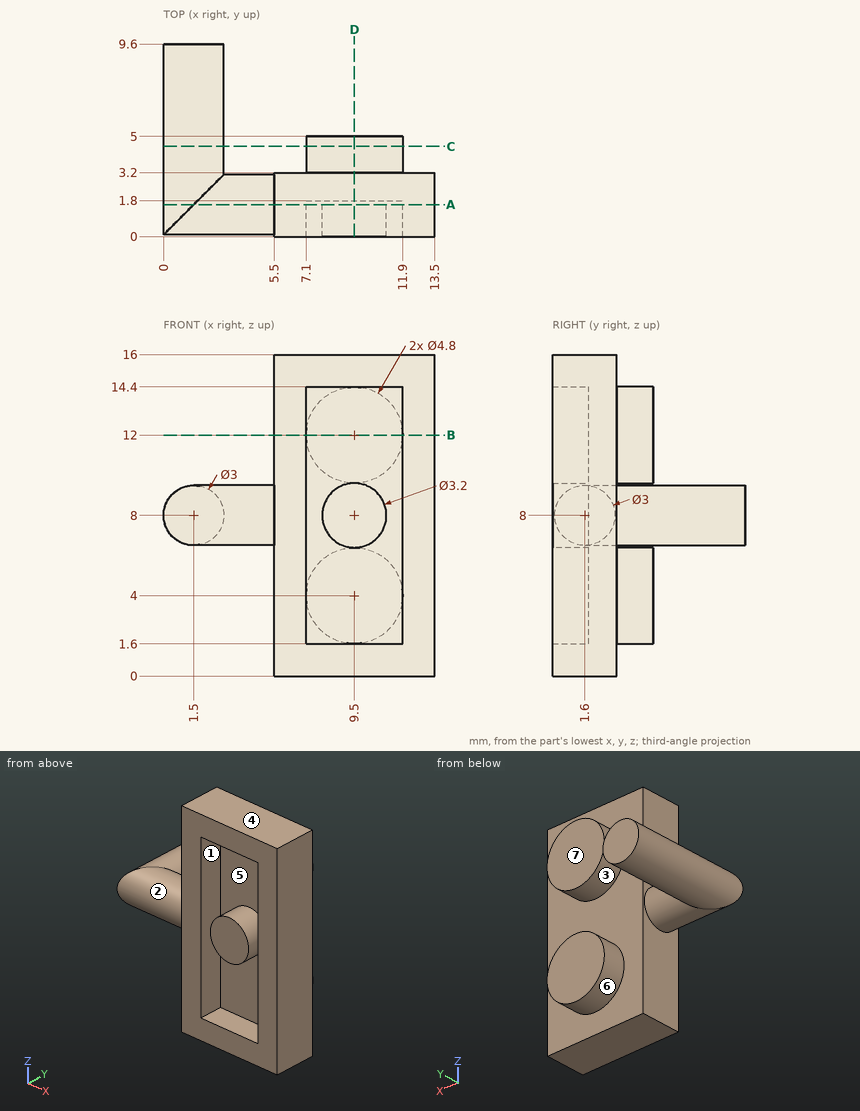
The drawing under review shows one solid part. Ordinate dimensions are in mm from its lowest x, y, z. A direction names the side the tool comes from. Round coordinates to 2 decimals unless told otherwise and drop trailing zeros. Loops run counter-clockwise (first coordinate to the right, second up) from the corner with the lowest first, then second, coordinate; pieces in that order, holes last. Notation, with made-up numbers: (61, -16) - (74, -16) arc R17 cw to (74, 3) - close; hole circle Ø5 at (-10.5, -18). An arc over 180 degrees is marked (long way). Put each result on its own line as item: value. Start each with the question number.
1. For the marked faces 5, 6 and 7, list the 3-axis set-ups (+Z, -Z, +X, -X, +Y, -Y) from which the entire face can be reached by the end or side of a thin tool; tool diameter is ignored.
2. Insertion check: P1, Ø1, axis at x = 4, z = 8.5, coming from the +Y side; P2, Ø1, axis at x = 3.5, z = 5.5, coming from the -Y side; P3, Ø4, axis at x = 5, z = 11, coming from the -Y side; P4, Ø2.5, axis at x = 10, z = 12, coming from the +Y side. Each pin has a flat end and moves straight along its axis. Give the tip position at first contact, or say it passes through.
3. Consider section C-C on y = 4.5. State the section outline as (x, z) points, plus the area to 3 significant figures.
4. Mouldability with a two-part tool opening along X and no side actions: class the marked faces 1, 2, 3 and 4 as +X half, -X half, draft (parallel to the pull), parting line (faces both ways), or undercut.
5. Consider section A-A on y = 1.6. State the section outline as (x, z) points.
6. Consider section B-B on z = 12. State the section outline as (x, y) points, plus the area to 3 significant figures.
7. Consider section D-D on x = 9.5. State the section outline as (y, z) points.
8. For probe 1 along Z at (x, y) = (10, 1.5); probe 2 along Y at (x, z) = (7, 10); probe 3 along X at (y, z) = (3, 4.5), list the stretches that pass through material, from the lowest coordinate up. Write a range as [from, to].
Result sheet:
1. face 5: -Y
1. face 6: +Y
1. face 7: +Z, -Z, +X, -X, +Y
2. P1: y = 3.1
2. P2: through
2. P3: y = 0
2. P4: y = 5
3. outline: circle Ø3 at (1.5, 8); circle Ø4.8 at (9.5, 4); circle Ø4.8 at (9.5, 12)
3. area: 43.3 mm^2
4. face 1: undercut
4. face 2: undercut
4. face 3: parting line
4. face 4: draft
5. outline: (1.5, 6.5) - (5.5, 6.5) - (5.5, 0) - (13.5, 0) - (13.5, 16) - (5.5, 16) - (5.5, 9.5) - (1.5, 9.5) arc R1.5 ccw to start; circle Ø3.2 at (9.5, 8); hole (7.1, 1.6) - (11.9, 1.6) - (11.9, 14.4) - (7.1, 14.4) - close
6. outline: (5.5, 0) - (7.1, 0) - (7.1, 1.8) - (11.9, 1.8) - (11.9, 0) - (13.5, 0) - (13.5, 3.2) - (11.9, 3.2) - (11.9, 5) - (7.1, 5) - (7.1, 3.2) - (5.5, 3.2) - close
6. area: 25.6 mm^2
7. outline: (0, 0) - (3.2, 0) - (3.2, 1.6) - (5, 1.6) - (5, 6.4) - (3.2, 6.4) - (3.2, 9.6) - (5, 9.6) - (5, 14.4) - (3.2, 14.4) - (3.2, 16) - (0, 16) - (0, 14.4) - (1.8, 14.4) - (1.8, 9.6) - (0, 9.6) - (0, 6.4) - (1.8, 6.4) - (1.8, 1.6) - (0, 1.6) - close
8. probe 1: [0, 1.6], [6.48, 9.52], [14.4, 16]
8. probe 2: [0, 3.2]
8. probe 3: [5.5, 13.5]
